Autodesk Inventor part; units mm, degrees
ref_plane "Work Plane1" through (40, 0, 0) normal (1, 0, 0) x (0, 1, 0)
ref_plane "XZ Plane" through (0, 0, 0) normal (0, 1, 0) x (-1, 0, 0)
ref_plane "XY Plane" through (0, 0, 0) normal (0, 0, 1) x (1, 0, 0)
sketch "Sketch1" plane through (0, 0, 0) normal (0, 1, 0) x (-1, 0, 0)
  line L0 (-60, -80) -> (60, -80)
  line L1 (80, -60) -> (80, 60)
  line L2 (60, 80) -> (-60, 80)
  line L3 (-80, 60) -> (-80, -60)
  line L4 (-80, -80) -> (80, 80) construction
  line L5 (80, -80) -> (-80, 80) construction
  arc A0 (80, 60) -> (60, 80) centre (60, 60) ccw
  arc A1 (-60, 80) -> (-80, 60) centre (-60, 60) ccw
  arc A2 (-80, -60) -> (-60, -80) centre (-60, -60) ccw
  arc A3 (60, -80) -> (80, -60) centre (60, -60) ccw
  point P0 (0, 0)
  dimension "d0" = 160
  dimension "d1" = 160
  dimension "d2" = 20
extrude "Extrusion1" add sketch "Sketch1" along normal blind 40
sketch "Sketch2" plane through (0, 0, 0) normal (0, -1, 0) x (1, 0, 0)
  line L0 (-55, -52.5) -> (55, 52.5) construction
  line L1 (55, -52.5) -> (-55, 52.5) construction
  line L2 (90.8825, 0) -> (-87.3629, 0)
  line L3 (0, 94.4084) -> (0, -106.3516)
  line L4 (-40, -60) -> (40, -60)
  line L5 (60, -40) -> (60, 40)
  line L6 (40, 60) -> (-40, 60)
  line L7 (-60, 40) -> (-60, -40)
  line L8 (-60, -60) -> (60, 60) construction
  line L9 (60, -60) -> (-60, 60) construction
  line L10 (60, 60) -> (41.9971, 60)
  line L11 (60, -60) -> (41.9971, -60)
  line L12 (60, 60) -> (60, 71.6594)
  line L13 (60, -60) -> (60, -69.6689)
  arc A0 (60, 40) -> (40, 60) centre (40, 40) ccw
  arc A1 (-40, 60) -> (-60, 40) centre (-40, 40) ccw
  arc A2 (-60, -40) -> (-40, -60) centre (-40, -40) ccw
  arc A3 (40, -60) -> (60, -40) centre (40, -40) ccw
  point P0 (0, 0)
  dimension "d23" = 60
  dimension "d25" = 60
  dimension "d26" = 20
extrude "Extrusion2" add sketch "Sketch2" along normal blind 40
sketch "Sketch3" plane through (0, 40, 0) normal (0, 1, 0) x (1, 0, 0)
  circle A0 centre (-37.5, -55) radius 5
  circle A1 centre (37.5, -55) radius 5
  line L0 (-35.6722, 52.5) -> (-19.5402, 52.5)
  line L1 (0, 83.5001) -> (0, -85.7722)
  line L2 (-75.2069, 0) -> (80.66, 0)
  line L3 (-37.5, -55) -> (37.5, -55)
  line L4 (-37.5, -55) -> (-37.5, -56.2391)
  line L5 (37.5, -55) -> (37.5, -56.2391)
  circle A2 centre (-37.5, 55) radius 5
  circle A3 centre (37.5, 55) radius 5
  point P0 (0, 0)
  dimension "d15" = 37.5
  dimension "d16" = 37.5
  dimension "d17" = 55
  dimension "d20" = 10
  dimension "d21" = 10
extrude "Extrusion3" cut sketch "Sketch3" against normal blind 6
ref_plane "Work Plane1" through (40, 0, 0) normal (1, 0, 0) x (0, 1, 0)
sketch "Sketch4" plane through (40, 0, 0) normal (1, 0, 0) x (0, 1, 0)
  arc A0 (-396.1638, 317.7429) -> (-418.612, 279.2134) centre (-410, 300) ccw
  circle A1 centre (-410, 300) radius 300
  line L0 (-40, -40) -> (-40, 40)
  line L1 (40, 60) -> (40, -60)
  line L2 (63.9503, 0) -> (-247.3631, 0)
  line L3 (-410, 300) -> (-214.4005, 300)
  line L4 (-40, -40) -> (-84.0453, -40)
  line L5 (-40, 40) -> (-40, -40)
  line L6 (-40, 40) -> (-396.1638, 317.7429)
  line L7 (-84.0453, -40) -> (-418.612, 279.2134)
  point P0 (0, 0)
  point P1 (-131.6551, 40.5657)
  dimension "d28" = 45
  dimension "d29" = 600
  dimension "d30" = 450
  dimension "d31" = 300
extrude "Extrusion4" add sketch "Sketch4" against normal blind 17.5 contours L6 A1 L7 A0 | A1 L6 L0 L2 L7 | L2 L0 L4 L7 picked at (-333.3289, 219.1483)
mirror "Mirror1" about plane through (0, 0, 0) normal (1, 0, 0) of "Extrusion4"
sketch "Sketch5" plane through (60, 0, 40) normal (1, 0, 0) x (0, 0, -1)
  arc A0 (-277.7429, -396.1638) -> (-239.2134, -418.612) centre (-260, -410) ccw
  circle A1 centre (-260, -410) radius 7.5
  point P0 (40, 0)
  dimension "d35" = 15
extrude "Extrusion5" cut sketch "Sketch5" against normal through all
properties part number "Plate2" material "Polyethylene, High Density"
Build history of the part. All positions in model axes, mm. A direction names the side the tool comes from. Round coordinates to 2 decimals unless told otherwise and drop trailing zeros. Order: outer loops, then holes, each group sorted by start corner. A loop starts at its lowest first (then second) coordinate and runs counter-clockwise, first axis right, second up. Notation, with made-up numbers: (-1, 34.5) - (57, 34.5) arc R19 ccw to (57, 71.5) - close; hole circle Ø2 at (-28, 66). An arc over 180 degrees is marked (long way). Use a Markdown table: item, result.
1) Flat gauge pins, fed straight in: pin 1 Ø11.5 at (x, z) = (37.5, 55) entering from -Y; pin 2 Ø5 at (x, z) = (-38.5, -53) entering from +Y; pin 3 Ø8 at (y, z) = (-299.5, 183.5) entering from -X. Where does each tip first touch, or does it go through?
Recorded:
| item | result |
|---|---|
| pin 1 | stops at y = -189.64 |
| pin 2 | stops at y = 34 |
| pin 3 | stops at x = -40 |
2) Saw through at B-B on z = 300. Write the cut outline in (x, y), and give its area (3 significant figures).
Recorded:
| item | result |
|---|---|
| outline | (-40, -432.5) - (-22.5, -432.5) - (-22.5, -417.5) - (-40, -417.5) - close; (-40, -402.5) - (-22.5, -402.5) - (-22.5, -373.41) - (-40, -373.41) - close; (22.5, -432.5) - (40, -432.5) - (40, -417.5) - (22.5, -417.5) - close; (22.5, -402.5) - (40, -402.5) - (40, -373.41) - (22.5, -373.41) - close |
| area | 1,540 mm² |
3) Saw through at C-C on x = -1. Write the cut outline in (y, z).
Recorded:
| item | result |
|---|---|
| outline | (-40, -60) - (0, -60) - (0, -80) - (40, -80) - (40, 80) - (0, 80) - (0, 60) - (-40, 60) - close |
4) Saw through at A-A on y = -340.5. Write the cut outline in (x, z).
Recorded:
| item | result |
|---|---|
| outline | (-40, 204.69) - (-22.5, 204.69) - (-22.5, 274.34) - (-40, 274.34) - close; (22.5, 204.69) - (40, 204.69) - (40, 274.34) - (22.5, 274.34) - close |
5) Pull direction Z, two halves, no side cores. Call faces 5 (the face through (-31.37, -253.67, 121.84)), 6 (the face through (60, -20, -1)), 7 (the face through (-38, 34, 55)), 8 (the face through (37, 34, 55)): pulls with the +Z half, pulls with the -Z half, needs draft (parallel to the pull), parting line crosses it, or undercut.
Recorded:
| item | result |
|---|---|
| face 5 | pulls with the -Z half |
| face 6 | needs draft |
| face 7 | undercut |
| face 8 | undercut |
6) Tool access for faces 1 (the face through (22.5, -208, 129)), 2 (the face through (31, -62, -40)), 3 (the face through (-40, -221, 129)), 4 (the face through (-54.297, -19.72, 53.986)): list every direction of +Z, -Z, +X, -X, +Y, -Y with a clear straight run to the whole face (end or side of a thin tool).
Recorded:
| item | result |
|---|---|
| face 1 | +Z, -Z, -Y |
| face 2 | -Z, +X, -X, -Y |
| face 3 | +Z, -Z, -X, -Y |
| face 4 | +Z, -X, -Y |
7) Wall check: L1, parallel to Z at x = 37.5, y = 37.9; L2, parallel to X at y = 36.65, z = 55; L3, parallel to X at y = -211, z = 95.5. Give the ranges that are in metal, low to high.
Recorded:
| item | result |
|---|---|
| L1 | z = -80 to -60, -50 to 50, 60 to 80 |
| L2 | x = -80 to -42.5, -32.5 to 32.5, 42.5 to 80 |
| L3 | x = -40 to -22.5, 22.5 to 40 |
8) Saw through at D-D on z = 157.5. Write the cut outline in (x, y).
Recorded:
| item | result |
|---|---|
| outline | (-40, -291.04) - (-22.5, -291.04) - (-22.5, -190.68) - (-40, -190.68) - close; (22.5, -291.04) - (40, -291.04) - (40, -190.68) - (22.5, -190.68) - close |
